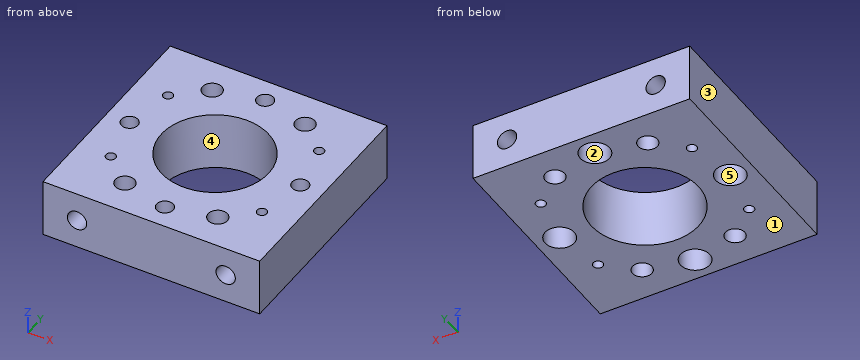
Autodesk Inventor part; units mm, degrees
ref_plane "YZ Plane" through (0, 0, 0) normal (1, 0, 0) x (0, 1, 0)
ref_plane "XZ Plane" through (0, 0, 0) normal (0, 1, 0) x (-1, 0, 0)
ref_plane "XY Plane" through (0, 0, 0) normal (0, 0, 1) x (1, 0, 0)
sketch "Sketch1" plane through (0, 0, 0) normal (0, 0, 1) x (1, 0, 0)
  line L0 (-22.225, 22.225) -> (22.225, 22.225)
  line L1 (22.225, 22.225) -> (22.225, -22.225)
  line L2 (22.225, -22.225) -> (-22.225, -22.225)
  line L3 (-22.225, -22.225) -> (-22.225, 22.225)
  line L4 (0, 0) -> (0, 22.225) construction
  line L5 (0, 0) -> (0, -22.225) construction
  line L6 (0, 0) -> (22.225, 0) construction
  line L7 (0, 0) -> (-22.225, 0) construction
  dimension "d0" = 44.45
  dimension "d1" = 44.45
extrude "Extrusion1" add sketch "Sketch1" along normal mid plane 11.938
sketch "Sketch2" plane through (0, 0, -5.969) normal (0, 0, -1) x (-1, 0, 0)
  point P0 (0, 0)
hole "Hole1" at (0, 0, -5.969) direction (0, 0, 1) diameter 22 end through all
sketch "Sketch3" plane through (0, 0, -5.969) normal (0, 0, -1) x (-1, 0, 0)
  circle A0 centre (0, 0) radius 11
  point P0 (0, 17.5)
  dimension "d11" = 17.5
hole "Hole2" at (0, 17.5, -5.969) direction (0, 0, 1) diameter 3.4 end through all counterbore diameter 6 counterbore depth 5.5
pattern_circular "Circular Pattern1" count 4 over 360 about axis through (0, 0, 58.0163) along (0, 0, -1) of "Hole2"
sketch "Sketch4" plane through (0, 0, -5.969) normal (0, 0, -1) x (-1, 0, 0)
  circle A0 centre (0, 0) radius 11
  circle A1 centre (0, 17.5) radius 3
  point P0 (-9.525, 15.24)
  dimension "d22" = 15.24
  dimension "d49" = 9.525
hole "Hole3" at (9.525, 15.24, -5.969) direction (0, 0, 1) diameter 3.962 end through all
mirror "Mirror1" about plane through (0, 0, 0) normal (1, 0, 0) of "Hole3"
mirror "Mirror2" about plane through (0, 0, 0) normal (0, 1, 0) of "Hole3", "Mirror1"
sketch "Sketch5" plane through (0, 0, -5.969) normal (0, 0, -1) x (-1, 0, 0)
  circle A0 centre (0, 0) radius 11
  point P0 (-15.5, 10)
  dimension "d31" = 10
  dimension "d32" = 15.5
hole "Hole4" at (15.5, 10, -5.969) direction (0, 0, 1) diameter 2.013 end through all
mirror "Mirror3" about plane through (0, 0, 0) normal (0, 1, 0) of "Hole4"
mirror "Mirror4" about plane through (0, 0, 0) normal (1, 0, 0) of "Hole4", "Mirror3", "Hole1"
sketch "Sketch6" plane through (-22.225, 22.225, 5.969) normal (0, 1, 0) x (1, 0, 0)
  line L0 (0, 0) -> (44.45, 0)
  line L1 (44.45, 11.938) -> (0, 11.938)
  line L2 (22.225, 0) -> (22.225, 11.938) construction
  line L3 (44.45, 0) -> (44.45, 11.938)
  line L4 (0, 11.938) -> (0, 0)
  line L5 (0, 5.969) -> (44.45, 5.969) construction
  point P0 (37.465, 5.969)
  dimension "d41" = 15.24
hole "Hole5" at (15.24, 22.225, 0) direction (0, -1, 0) diameter 3.962 depth 6 tip angle 118
mirror "Mirror5" about plane through (0, 0, 0) normal (1, 0, 0) of "Hole5"
mirror "Mirror6" about plane through (0, 0, 0) normal (0, 1, 0) of "Hole5", "Mirror5"
properties part number "BB1-FrontPlate" material "Steel, Mild"
Part model, mm, in its own coordinate system. Face numbers are marked on the shaded views. A direction names the side the tool comes from. Round coordinates to 2 decimals unless told otherwise and drop trailing zeros. Write each loop counter-clockwise with the first axis right and the second up, starting at its lowest first coordinate (ties: lowest second). Pieces come first, ordered by that corner, then holes. Notation, with made-up numbers: M 15.25,59.5 L 59.25,59.5 A26 ccw 59.25,77.5 Z; hole C 6.5,-7.75 d10. An arc over 180 degrees is marked long. One line per question, with ' | ' between items.
(1) Saw through at B-B on x = 4. Write the cut outline in (y, z) (3 decimals), then the cut area to 3 significant figures.
Answer key:
outline: M -22.225,-5.969 L -10.247,-5.969 L -10.247,5.969 L -22.225,5.969 Z; M 10.247,-5.969 L 22.225,-5.969 L 22.225,5.969 L 10.247,5.969 Z | area: 286 mm^2
(2) Probe line 1 along X through (y, z) = (-15.24, 1.25) (3 decimals); line 2 along X through (y, z) = (-17.5, 4) (3 decimals); line 3 along X through (y, z) = (-8, -3.75) (3 decimals). List the from-to ranges inside material, lowest first.
Answer key:
line 1: x = -22.225 to -11.506, -7.544 to 7.544, 11.506 to 22.225 | line 2: x = -22.225 to -1.7, 1.7 to 22.225 | line 3: x = -22.225 to -7.55, 7.55 to 22.225
(3) Saw through at C-C on z = 4. Count the separate pieces of the cut face and the enclosed holes in it, then the cut area to 3 significant figures.
Answer key:
separate pieces: 1 | enclosed holes: 13 | area: 1,500 mm^2
(4) Two-plate mould, pull along X, no slides. Class the marked faces 1, 2 and 3: released by +X, released by -X, zero draft, split by the parting line, or undercut.
Answer key:
face 1: zero draft | face 2: undercut | face 3: released by -X
(5) Pin check, flat tip, straight feed: pin 1 (3 mm diameter, centred on x = -0.5, y = 18.5, fed in from -Z). Stop position of the tip, or through.
Answer key:
pin 1: stops at z = -0.47
(6) 3-axis set-ups, long thin cutter, end or side, ignore diameter. For the marked faces 4 and 5: which of +Z, -Z, +X, -X, +Y, -Y reach the whole face in a straight line?
Answer key:
face 4: +Z, -Z | face 5: -Z
(7) Saw through at D-D on y = 6. Write the cut outline in (x, z) (3 decimals).
Answer key:
outline: M -22.225,-5.969 L -9.22,-5.969 L -9.22,5.969 L -22.225,5.969 Z; M 9.22,-5.969 L 22.225,-5.969 L 22.225,5.969 L 9.22,5.969 Z
(8) Saw through at A-A on y = 0. Write the cut outline in (x, z) (3 decimals), then the cut area to 3 significant figures.
Answer key:
outline: M -22.225,-5.969 L -20.5,-5.969 L -20.5,-0.469 L -19.2,-0.469 L -19.2,5.969 L -22.225,5.969 Z; M -15.8,-0.469 L -14.5,-0.469 L -14.5,-5.969 L -11,-5.969 L -11,5.969 L -15.8,5.969 Z; M 11,-5.969 L 14.5,-5.969 L 14.5,-0.469 L 15.8,-0.469 L 15.8,5.969 L 11,5.969 Z; M 19.2,-0.469 L 20.5,-0.469 L 20.5,-5.969 L 22.225,-5.969 L 22.225,5.969 L 19.2,5.969 Z | area: 158 mm^2
